The model under review builds one solid part; all positions refer to its coordinate system, in mm. A direction names the side the tool comes from. Coordinates: 2 decimals unless noted, no trailing zeros. Loops run counter-clockwise (first coordinate to the right, second up) from the corner with the lowest first, then second, coordinate; pieces in that order, holes last. Notation, with made-up numbers: M 70,22 L 96,22 A29 cw 96,51 Z; hole C -0.75,-22 d9. An arc over 180 degrees is marked long. Write item = value, one per line. Start each with the question number.
Q1. Mouldability with a two-part tool opening along Z and no side actions: class faces 3 (the face through (45.31, 0.88, 19.98)), 4 (the face through (13.76, -13.63, -8.41)), 5 (the face through (62.675, 14.334, -9.139)) as released by +Z, released by -Z, zero draft, split by the parting line, or undercut.
Q2. We need section A-A on y = -7. Give the boundary of the cut face in (x, z) (3 decimals), and give its area (3 significant figures).
Q3. We need section D-D on x = 51. Give the boundary of the cut face in (y, z).
Q4. Clearance check with flat-ended pins moving along their axes: pin 1 Ø1.5 at (x, z) = (57.5, 10) entering from +Y; pin 2 Ø1 at (x, z) = (19.5, -11.5) entering from +Y; pin 3 Ø4 at (x, z) = (61, 13.5) entering from +Y; pin 4 Ø2 at (y, z) = (8.5, -8.5) entering from -X. State where each tip first meets the part, or that it passes through.
Q5. Wall thickness on probe 1 along Y at (x, z) = (67.25, 0); probe 2 along Y at (x, z) = (20, 0): over which ranges is each line inside the solid? List them lowest first.
Q6. We need section B-B on z = 0. Give the boundary of the cut face in (x, y).
Q7. We need section C-C on x = 37. Give the boundary of the cut face in (y, z).
Q8. For faces 1 (the face through (75, -15, 9)), 2 (the face through (50, 8, -13)), list the 3-axis set-ups (+Z, -Z, +X, -X, +Y, -Y) from which the entire face can be reached by the end or side of a thin tool; tool diameter is ignored.
from build123d import *

# Parameters (mm, degrees)
SKETCH1_R               = 20
BOSS_EXTRUDE1_DEPTH     = 75
CUT_EXTRUDE2_DEPTH      = 81.156097709
CUT_EXTRUDE2_DEPTH_BACK = 81.156097709
SKETCH3_R               = 14.5
SKETCH4_R               = 17
CUT_EXTRUDE3_DEPTH      = 25
CUT_EXTRUDE4_DEPTH      = 81.156097709
CUT_EXTRUDE4_DEPTH_BACK = 81.156097709
SKETCH5_R               = 426.5


with BuildPart() as part:
    # Sketch1 → Boss-Extrude1 (new body)
    with BuildSketch(Plane(origin=(0, 0, 0), x_dir=(0, 0, -1), z_dir=(1, 0, 0))):
        Circle(SKETCH1_R)
    extrude(amount=BOSS_EXTRUDE1_DEPTH)

    # Sketch3 → Cut-Extrude2 (cut, two sides: drawn at the far end of the back side and taken through both)
    with BuildSketch(Plane(origin=(75, 0, 0), x_dir=(0, 0, -1), z_dir=(1, 0, 0)).offset(-CUT_EXTRUDE2_DEPTH_BACK)):
        Circle(SKETCH3_R)
    extrude(amount=CUT_EXTRUDE2_DEPTH + CUT_EXTRUDE2_DEPTH_BACK, mode=Mode.SUBTRACT)

    # Sketch4 → Cut-Extrude3 (cut)
    with BuildSketch(Plane(origin=(75, 0, 0), x_dir=(0, 0, -1), z_dir=(1, 0, 0))):
        Circle(SKETCH4_R)
    extrude(amount=-CUT_EXTRUDE3_DEPTH, mode=Mode.SUBTRACT)

    # Sketch5 → Cut-Extrude4 (cut, two sides: drawn at the far end of the back side and taken through both)
    with BuildSketch(Plane(origin=(0, 0, 0), x_dir=(1, 0, 0), z_dir=(0, 1, 0)).offset(-CUT_EXTRUDE4_DEPTH_BACK)):
        with Locations((-376.699150517, 180)):
            Circle(SKETCH5_R)
    extrude(amount=CUT_EXTRUDE4_DEPTH + CUT_EXTRUDE4_DEPTH_BACK, mode=Mode.SUBTRACT)


solid = part.part
Returned:
q1.face_3 = split by the parting line
q1.face_4 = released by -Z
q1.face_5 = undercut
q2.outline = M 0.669,18.735 A426.5 cw 3.787,12.698 L 50,12.698 L 50,15.492 L 75,15.492 L 75,18.735 Z; M 15.618,-12.698 A426.5 cw 18.137,-18.735 L 75,-18.735 L 75,-15.492 L 50,-15.492 L 50,-12.698 Z
q2.area = 650 mm^2
q3.outline = C 0,0 d40; hole C 0,0 d34
q4.pin_1 = 17.73
q4.pin_2 = 16.7
q4.pin_3 = 16.36
q4.pin_4 = through
q5.probe_1 = -20 to -17, 17 to 20
q5.probe_2 = -20 to -14.5, 14.5 to 20
q6.outline = M 9.96,-20 L 75,-20 L 75,-17 L 50,-17 L 50,-14.5 L 9.96,-14.5 Z; M 9.96,14.5 L 50,14.5 L 50,17 L 75,17 L 75,20 L 9.96,20 Z
q7.outline = C 0,0 d40; hole C 0,0 d29
q8.face_1 = +Z, -Z, +X, +Y, -Y
q8.face_2 = +X
